```python
from build123d import *

# Parameters (mm, degrees)
F0_W     = 200
F0_H     = 10
F1_DEPTH = 10
F3_D     = 6.35
F5_D     = 6.35
F7_D     = 6.35


with BuildPart() as f1:
    # F0 (on Front) → F1 (new body)
    with BuildSketch(Plane.XZ):
        with Locations((-50.903185, -11.052803)):
            Rectangle(F0_W, F0_H)
    extrude(amount=F1_DEPTH)

    # F3 (through all)
    with Locations(Plane.XZ.offset(10)):
        with Locations((-142.013185, -11.052803)):
            Hole(F3_D / 2)

    # F5 (through all)
    with Locations(Plane.XZ.offset(10)):
        with Locations((40.206815, -11.052803)):
            Hole(F5_D / 2)

    # F7 (through all)
    with Locations(Plane.XZ.offset(10)):
        with Locations((-50.903185, -11.052803)):
            Hole(F7_D / 2)


solid = f1.part
```
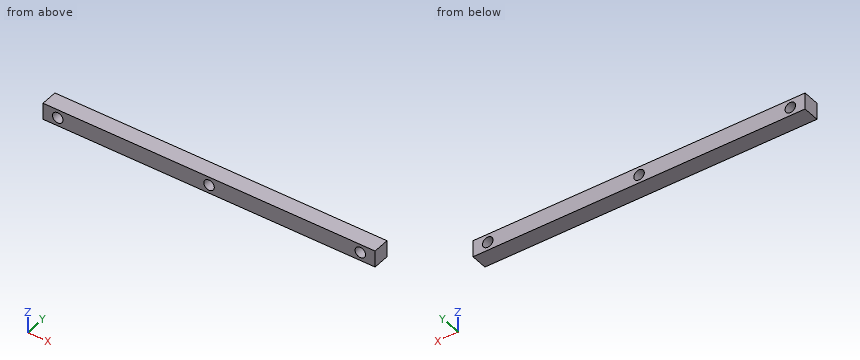
Check sheet for the modelled part. Datum: model origin and axes. Units: mm. Coordinates: 2 decimals unless noted, no trailing zeros. Write each loop counter-clockwise with the first axis right and the second up, starting at its lowest first coordinate (ties: lowest second). Pieces come first, ordered by that corner, then holes. Notation, with made-up numbers: (65.25, 31.25) -> (80.25, 31.25) arc R26 cw to (80.25, 49.25) -> close; hole circle Ø10 at (16.5, -5.5). An arc over 180 degrees is marked (long way). Use a Markdown table: item, result.
1. Sectioned sample at B-B (z = -9.5). Enter the section's corners in (x, y).
Reported:
| item | result |
|---|---|
| outline | (-150.9, -10) -> (-144.78, -10) -> (-144.78, 0) -> (-150.9, 0) -> close; (-139.24, -10) -> (-53.67, -10) -> (-53.67, 0) -> (-139.24, 0) -> close; (-48.13, -10) -> (37.44, -10) -> (37.44, 0) -> (-48.13, 0) -> close; (42.98, -10) -> (49.1, -10) -> (49.1, 0) -> (42.98, 0) -> close |
2. Scan lines: line 1 along X through (y, z) = (-3.75, -10.75); line 2 along X through (y, z) = (-5.5, -9.5); line 3 along Z through (x, y) = (-48, -5.5). Record each from-to range of solid material in increasing order.
Reported:
| item | result |
|---|---|
| line 1 | x = -150.9 to -145.17, -138.85 to -54.06, -47.74 to 37.05, 43.37 to 49.1 |
| line 2 | x = -150.9 to -144.78, -139.24 to -53.67, -48.13 to 37.44, 42.98 to 49.1 |
| line 3 | z = -16.05 to -12.34, -9.77 to -6.05 |
3. Go/stop test with a flat-tipped pin: pin 1 Ø5.5 at (x, z) = (-142.01, -11.05) entering from +Y. Record where the tip stops, or that it passes through.
Reported:
| item | result |
|---|---|
| pin 1 | passes through |
4. Sectioned sample at A-A (y = -7.5). Enter the section's corners in (x, z) (3 decimals), plus the area to 3 significant figures.
Reported:
| item | result |
|---|---|
| outline | (-150.903, -16.053) -> (49.097, -16.053) -> (49.097, -6.053) -> (-150.903, -6.053) -> close; hole circle Ø6.35 at (-142.013, -11.053); hole circle Ø6.35 at (-50.903, -11.053); hole circle Ø6.35 at (40.207, -11.053) |
| area | 1,900 mm2 |
